Could you check a few things on this model? Use its own coordinates, in mm. A direction names the side the tool comes from. Give positions to 0.01 mm unless a question says otherwise; leave off trailing zeros. Write each loop counter-clockwise with the first axis right and the second up, starting at its lowest first coordinate (ties: lowest second). Pieces come first, ordered by that corner, then holes. Notation, with made-up numbers: (49.25, 13.25) - (54.25, 13.25) arc R25 ccw to (54.25, 45.25) - close; hole circle Ø4 at (-17, 7). An arc over 180 degrees is marked (long way). Answer as CSV lines item,"result". Start each with the question number.
Q1. If I drill on line 1 along X through (y, z) = (11.9, 4) (3 decimals); line 2 along Z through (x, y) = (19, 6.5); line 3 along Z through (x, y) = (0, 7.5), over which ranges is the centre line in solid material (lowest first)?
Q2. Imagine slicing it at A-A on x = 19. List the corners of the cut face in (y, z) for me (3 decimals).
Q3. We'd pull the mould along Z, two halves only. Please class faces 3 (the face through (19, -4, 4)), 4 (the face through (0, 0, 138)), 5 (the face through (0, -12.5, 68)), 6 (the face through (-19, -4, 4)): pulls with the +Z half, pulls with the -Z half, needs draft (parallel to the pull), parting line crosses it, or undercut.
Q4. Will these pins go through, and if not, where does the flat tip stop? pin 1 Ø1.5 at (x, z) = (19.5, 4) entering from +Y; pin 2 Ø3 at (x, z) = (19.5, 5) entering from +Y; pin 3 Ø4.5 at (x, z) = (19, 4) entering from +Y.
Q5. On a 3-axis mill with a long thin cutter (end or side, diameter ignored), from which of +Z, -Z, +X, -X, +Y, -Y can I reach the whole of each face in a straight line? I mean faces 1 (the face through (-16.621, 12.007, 4.986)), 2 (the face through (0, 12.5, 68)). Say none if no direction works.
```python
from build123d import *

# Parameters (mm, degrees)
SKETCH2_W           = 46
SKETCH2_H           = 25
BOSS_EXTRUDE1_DEPTH = 138
SKETCH3_R           = 2.575
SKETCH3_R_2         = 1.25
CUT_EXTRUDE1_DEPTH  = 1
SKETCH4_R           = 2
SKETCH4_R_2         = 1
CUT_EXTRUDE2_DEPTH  = 16.5


with BuildPart() as part:
    # Sketch2 → Boss-Extrude1 (new body)
    with BuildSketch(Plane.XY):
        Rectangle(SKETCH2_W, SKETCH2_H)
    extrude(amount=BOSS_EXTRUDE1_DEPTH)

    # Sketch3 → Cut-Extrude1 (cut)
    with BuildSketch(Plane(origin=(0, 12.5, 0), x_dir=(1, 0, 0), z_dir=(0, 1, 0))):
        with Locations((-19, -4)):
            Circle(SKETCH3_R)
        with Locations((0, -5)):
            Circle(SKETCH3_R_2)
        with Locations((19, -4)):
            Circle(SKETCH3_R)
    extrude(amount=-CUT_EXTRUDE1_DEPTH, mode=Mode.SUBTRACT)

    # Sketch4 → Cut-Extrude2 (cut)
    with BuildSketch(Plane(origin=(0, 12.5, 0), x_dir=(1, 0, 0), z_dir=(0, 1, 0))):
        with Locations((-19, -4)):
            Circle(SKETCH4_R)
        with Locations((19, -4)):
            Circle(SKETCH4_R)
        with Locations((0, -5)):
            Circle(SKETCH4_R_2)
    extrude(amount=-CUT_EXTRUDE2_DEPTH, mode=Mode.SUBTRACT)


solid = part.part
```
Conclusion:
1,line 1,"-23 to -21.575, -16.425 to -0.75, 0.75 to 16.425, 21.575 to 23"
1,line 2,"0 to 2, 6 to 138"
1,line 3,"0 to 4, 6 to 138"
2,outline,"(-12.5, 0) - (12.5, 0) - (12.5, 1.425) - (11.5, 1.425) - (11.5, 2) - (-4, 2) - (-4, 6) - (11.5, 6) - (11.5, 6.575) - (12.5, 6.575) - (12.5, 138) - (-12.5, 138) - close"
3,face 3,"undercut"
3,face 4,"pulls with the +Z half"
3,face 5,"needs draft"
3,face 6,"undercut"
4,pin 1,"y = -4"
4,pin 2,"y = 12.5"
4,pin 3,"y = 11.5"
5,face 1,"+Y"
5,face 2,"+Z, -Z, +X, -X, +Y"
